Geometry check sheet. Reference: the model listing, model coordinates, mm. A direction names the side the tool comes from. Round coordinates to 2 decimals unless told otherwise and drop trailing zeros. Order: outer loops, then holes, each group sorted by start corner. A loop starts at its lowest first (then second) coordinate and runs counter-clockwise, first axis right, second up.
(1) Sectioned sample at C-C (z = 1.25). Record the boundary of the cut face in (x, y).
(2) Set-up check for faces 4 (the face through (26.024, -7.614, 9.914)), 5 (the face through (10.1, -12.5, -1.8)), 6 (the face through (11, 0, 12)), 7 (the face through (26, -14, 3)): record each of +Z, -Z, +X, -X, +Y, -Y from which the full face is reachable in a straight line by a thin tool's end or side.
(3) Material ranges on line 1 along X through (y, z) = (9, -5.25); line 2 along Z through (x, y) = (25.5, 0.5); line 3 along Z through (x, y) = (23.75, 0), recorded low to high.
(4) Release check for a two-part mould opening along Z. For faces 1 (the face through (0, -11, 0)), 2 (the face through (15, -7, 15)), 3 (the face through (26.02, -7.8, -9.77)) record: +Z half, -Z half, draft (parallel to the pull), parting line (faces both ways), or undercut.
(5) Go/stop test with flat-tipped pins: pin 1 (2 mm diameter, centred on x = 24.5, y = 6.5, fed in from -Z); pin 2 (12 mm diameter, centred on x = 9.5, z = -10.5, fed in from +Y); pin 3 (6.5 mm diameter, centred on x = 13, z = -1, fed in from -Y); pin 4 (5 mm diameter, centred on x = 12.5, z = 0, fed in from -Y). Record where each tip stops, or that it passes through.
(6) Sectioned sample at D-D (x = 19.5). Record the boundary of the cut face in (y, z).
(7) Sectioned sample at B-B (y = 4.5). Record the boundary of the cut face in (x, z), plus the area to 3 significant figures.
Autodesk Inventor part; units mm, degrees
ref_plane "YZ Plane" through (0, 0, 0) normal (1, 0, 0) x (0, 1, 0)
ref_plane "XZ Plane" through (0, 0, 0) normal (0, 1, 0) x (-1, 0, 0)
ref_plane "XY Plane" through (0, 0, 0) normal (0, 0, 1) x (1, 0, 0)
sketch "スケッチ1" plane through (0, 0, 0) normal (1, 0, 0) x (0, 1, 0)
  line L0 (-15, 0) -> (-15, 15)
  line L1 (-15, 15) -> (0, 15)
  line L2 (-15, 0) -> (-15, -15)
  line L3 (-15, -15) -> (0, -15)
  arc A0 (0, -15) -> (0, 15) centre (0, 0) ccw
  dimension "d0" = 15
  dimension "d1" = 15
  dimension "d2" = 15
  dimension "d3" = 15
  dimension "d4" = 30
extrude "押し出し1" add sketch "スケッチ1" along normal blind 30
sketch "スケッチ2" plane through (30, 0, 0) normal (1, 0, 0) x (0, 0, -1)
  circle A0 centre (0, 0) radius 9
  dimension "d7" = 18
extrude "押し出し2" cut sketch "スケッチ2" against normal blind 7.5
sketch "スケッチ3" plane through (22.5, 0, 0) normal (1, 0, 0) x (0, 0, -1)
  circle A0 centre (0, 0) radius 12.7
  dimension "d10" = 25.4
extrude "押し出し3" cut sketch "スケッチ3" against normal blind 6
sketch "スケッチ4" plane through (16.5, 0, 0) normal (1, 0, 0) x (0, 0, -1)
  circle A0 centre (0, 0) radius 10
  dimension "d13" = 20
extrude "押し出し4" cut sketch "スケッチ4" against normal through all
sketch "スケッチ5" plane through (0, 0, 0) normal (-1, 0, 0) x (0, 0, 1)
  arc A0 (15, 0) -> (-15, 0) centre (0, 0) ccw
  line L0 (-15, 0) -> (15, 0)
  dimension "d16" = 30
extrude "押し出し5" cut sketch "スケッチ5" against normal blind 22.5
sketch "スケッチ6" plane through (30, 0, 0) normal (1, 0, 0) x (0, 0, -1)
  arc A0 (-12.5, 0) -> (12.5, 0) centre (0, 0) ccw
  arc A1 (15, 0) -> (-15, 0) centre (0, 0) ccw
  line L0 (-12.5, 0) -> (12.5, 0)
  line L1 (12.5, 0) -> (12.5, 20)
  line L2 (12.5, 20) -> (-12.5, 20)
  line L3 (-12.5, 20) -> (-12.5, 0)
  point P0 (12.5, 8.2916)
  point P1 (-12.5, 8.2916)
  dimension "d19" = 25
  dimension "d20" = 25
  dimension "d21" = 20
extrude "押し出し6" cut sketch "スケッチ6" against normal blind 5.75 contours L0 A0 | L3 A1 L1 L0
sketch "スケッチ7" plane through (30, 0, 0) normal (1, 0, 0) x (0, 0, -1)
  arc A0 (-12.5, 0) -> (12.5, 0) centre (0, 0) ccw
  arc A1 (15, 0) -> (-15, 0) centre (0, 0) ccw
  line L0 (-15, 0) -> (15, 0)
  dimension "d24" = 25
  dimension "d25" = 30
extrude "押し出し7" add sketch "スケッチ7" against normal blind 2.25
sketch "スケッチ8" plane through (30, 0, 0) normal (1, 0, 0) x (0, 0, -1)
  circle A0 centre (0, 0) radius 9
  dimension "d28" = 18
extrude "押し出し8" cut sketch "スケッチ8" against normal through all
sketch "スケッチ9" plane through (0, -15, -15) normal (0, -1, 0) x (1, 0, 0)
  line L0 (0, 15) -> (26, 15) construction
  line L1 (27.75, 12) -> (24.25, 12)
  line L2 (24.25, 12) -> (24.25, 18)
  line L3 (24.25, 18) -> (27.75, 18)
  line L4 (27.75, 18) -> (27.75, 12)
  line L5 (27.75, 12) -> (24.25, 18) construction
  line L6 (24.25, 12) -> (27.75, 18) construction
  dimension "d31" = 26
  dimension "d32" = 3.5
  dimension "d33" = 6
extrude "押し出し9" cut sketch "スケッチ9" against normal through all
sketch "スケッチ10" plane through (0, -15, -15) normal (0, -1, 0) x (1, 0, 0)
  line L0 (0, 15) -> (12.5, 15) construction
  circle A0 centre (12.5, 15) radius 3
  dimension "d36" = 12.5
  dimension "d37" = 6
extrude "押し出し10" cut sketch "スケッチ10" against normal blind 5
thread "ねじ1"
fillet "フィレット1" radius 2 2 edges at (15, -15, -15) (15, -15, 15)
properties part number "コリメータマウント"
Answer below:
1. outline: (0, -15) - (9.77, -15) - (9.77, -10) - (15.23, -10) - (15.23, -15) - (24.25, -15) - (24.25, -8.91) - (22.5, -8.91) - (22.5, -12.64) - (16.5, -12.64) - (16.5, -9.92) - (0, -9.92) - close; (22.5, 8.91) - (24.25, 8.91) - (24.25, 14.95) - (22.5, 14.95) - close; (27.75, -15) - (30, -15) - (30, -8.91) - (27.75, -8.91) - close; (27.75, 8.91) - (30, 8.91) - (30, 14.95) - (27.75, 14.95) - close
2. face 4: +Y
2. face 5: -Y
2. face 6: +Z, -Z, -X, +Y
2. face 7: +Y, -Y
3. line 1: x = 22.5 to 24.25, 27.75 to 30
3. line 2: z = -14.99 to -12.5, 12.5 to 14.99
3. line 3: z = -15 to -9, 9 to 15
4. face 1: draft
4. face 2: +Z half
4. face 3: undercut
5. pin 1: stops at z = -13.96
5. pin 2: stops at y = 0
5. pin 3: stops at y = -15
5. pin 4: stops at y = -10
6. outline: (-15, -13) arc R2 ccw to (-13, -15) - (0, -15) - (0, -12.7) arc R12.7 cw to (0, 12.7) - (0, 15) - (-13, 15) arc R2 ccw to (-15, 13) - close
7. outline: (22.5, -14.31) - (30, -14.31) - (30, -7.79) - (27.75, -7.79) - (27.75, -12.5) - (24.25, -12.5) - (24.25, -7.79) - (22.5, -7.79) - close; (22.5, 7.79) - (24.25, 7.79) - (24.25, 12.5) - (27.75, 12.5) - (27.75, 7.79) - (30, 7.79) - (30, 14.31) - (22.5, 14.31) - close
7. area: 64.8 mm2
